Can you work these out from the model? Positions are in its coordinate system, mm. Face numbers are marked on the shaded views. A direction names the side the tool comes from. Coordinates: 2 decimals unless noted, no trailing zeros. Order: outer loops, then holes, each group sorted by start corner. A loop starts at its lowest first (then second) coordinate and runs counter-clockwise, first axis right, second up. Notation, with made-up numbers: M 46,-34 L 67,-34 A10 ccw 67,-23 Z; hole C 35,-22.75 d3. An arc over 180 degrees is marked long. Answer as a JSON object with one key per item and string values.
from build123d import *

# Parameters (mm, degrees)
SKETCH_4_W          = 28.4
SKETCH_4_H          = 61.796304386
EXTRUDE_1_DEPTH     = 5
CUT_EXTRUDE_START   = 5
SKETCH_4_4_R        = 3.1
CUT_EXTRUDE_1_DEPTH = 2.6
SKETCH_4_5_R        = 2
CUT_EXTRUDE_2_DEPTH = 74.193425166
SKETCH_4_6_W        = 13.4
SKETCH_4_6_H        = 41.796304386
CUT_EXTRUDE_3_DEPTH = 69.193425166
SKETCH_5_W          = 5
SKETCH_5_H          = 20
EXTRUDE_2_DEPTH     = 4
SKETCH_5_3_R        = 1.5
CUT_EXTRUDE_5_DEPTH = 69.193425166
CUT_EXTRUDE_START_2 = 4
SKETCH_5_4_R        = 2.25
CUT_EXTRUDE_7_DEPTH = 2


with BuildPart() as part:
    # 草图4 → 凸台-拉伸1 (new body)
    with BuildSketch(Plane(origin=(0, 0, 0), x_dir=(1, 0, 0), z_dir=(0, 1, 0))):
        with Locations((-14.2, -30.898152193)):
            Rectangle(SKETCH_4_W, SKETCH_4_H)
    extrude(amount=EXTRUDE_1_DEPTH)

    # 草图4<4> → 切除-拉伸1 (cut)
    with BuildSketch(Plane(origin=(0, 0, 0), x_dir=(1, 0, 0), z_dir=(0, 1, 0)).offset(CUT_EXTRUDE_START)):
        with Locations(Location((-13.9, -13.4, 0), (0, 0, 90))):
            Circle(SKETCH_4_4_R)
        with Locations(Location((-23.4, -34.346360066, 0), (0, 0, 90))):
            Circle(SKETCH_4_4_R)
        with Locations(Location((-18.4, -56.796304386, 0), (0, 0, 90))):
            Circle(SKETCH_4_4_R)
    extrude(amount=-CUT_EXTRUDE_1_DEPTH, mode=Mode.SUBTRACT)

    # 草图4<5> → 切除-拉伸2 (cut, through all)
    with BuildSketch(Plane(origin=(0, 0, 0), x_dir=(1, 0, 0), z_dir=(0, 1, 0)).offset(CUT_EXTRUDE_START)):
        with Locations(Location((-13.9, -13.4, 0), (0, 0, 90))):
            Circle(SKETCH_4_5_R)
        with Locations(Location((-23.4, -34.346360066, 0), (0, 0, 90))):
            Circle(SKETCH_4_5_R)
        with Locations(Location((-18.4, -56.796304386, 0), (0, 0, 90))):
            Circle(SKETCH_4_5_R)
    extrude(amount=-CUT_EXTRUDE_2_DEPTH, mode=Mode.SUBTRACT)

    # 草图4<6> → 切除-拉伸3 (cut, through all)
    with BuildSketch(Plane(origin=(0, 0, 0), x_dir=(1, 0, 0), z_dir=(0, 1, 0))):
        with Locations((-6.7, -40.898152193)):
            Rectangle(SKETCH_4_6_W, SKETCH_4_6_H)
    extrude(amount=CUT_EXTRUDE_3_DEPTH, mode=Mode.SUBTRACT)

    # 草图5 → 凸台-拉伸2 (add)
    with BuildSketch(Plane.XZ):
        Polygon((5, -10), (5, 20), (-28.4, 20), (-28.4, -10), (0, -10), align=None)
        with Locations((2.5, -20)):
            Rectangle(SKETCH_5_W, SKETCH_5_H)
    extrude(amount=EXTRUDE_2_DEPTH)

    # 草图5<3> → 切除-拉伸5 (cut, through all)
    with BuildSketch(Plane.XZ):
        with Locations(Location((-17.4, -5, 0), (0, 0, 270))):
            Circle(SKETCH_5_3_R)
        with Locations(Location((-5, -5, 0), (0, 0, 270))):
            Circle(SKETCH_5_3_R)
        with Locations(Location((2.5, 10, 0), (0, 0, 270))):
            Circle(SKETCH_5_3_R)
        with Locations(Location((2.5, -20, 0), (0, 0, 270))):
            Circle(SKETCH_5_3_R)
    extrude(amount=CUT_EXTRUDE_5_DEPTH, mode=Mode.SUBTRACT)

    # 草图5<4> → 切除-拉伸7 (cut)
    with BuildSketch(Plane.XZ.offset(CUT_EXTRUDE_START_2)):
        with Locations(Location((-17.4, -5, 0), (0, 0, 270))):
            Circle(SKETCH_5_4_R)
        with Locations(Location((-5, -5, 0), (0, 0, 270))):
            Circle(SKETCH_5_4_R)
        with Locations(Location((2.5, 10, 0), (0, 0, 270))):
            Circle(SKETCH_5_4_R)
        with Locations(Location((2.5, -20, 0), (0, 0, 270))):
            Circle(SKETCH_5_4_R)
    extrude(amount=-CUT_EXTRUDE_7_DEPTH, mode=Mode.SUBTRACT)


solid = part.part
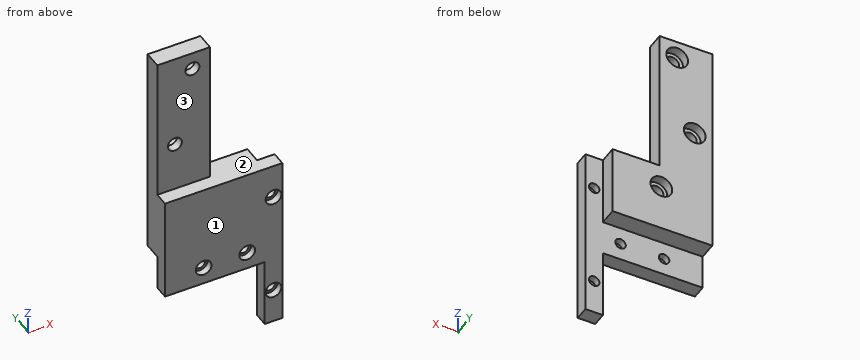
Item 1: I'm going to push flat-ended pins straight in: pin 1 (3 mm diameter, centred on x = -13, z = 14, fed in from +Y); pin 2 (2.5 mm diameter, centred on y = 1.5, z = 44.5, fed in from +X); pin 3 (1.2 mm diameter, centred on x = -14.5, z = 14, fed in from +Y). Where does each tip first touch, or does it pass through?
Answers follow:
{"pin 1": "stops at y = 2.4", "pin 2": "stops at x = -13.4", "pin 3": "stops at y = 0"}
Item 2: I want a section at D-D, the plane z = 40. Write out the boundary of the cut face in (x, y), plus the area to 3 significant figures.
Answers follow:
{"outline": "M -28.4,0 L -13.4,0 L -13.4,5 L -28.4,5 Z", "area": "75.0 mm^2"}
Item 3: I want a section at B-B, the plane y = 1. Write out the boundary of the cut face in (x, z), plus the area to 3 significant figures.
Answers follow:
{"outline": "M -28.4,0 L 0,0 L 0,20 L -13.4,20 L -13.4,61.8 L -28.4,61.8 Z; hole C -23.4,34.35 d4; hole C -18.4,56.8 d4; hole C -13.9,13.4 d4", "area": "1,160 mm^2"}
Item 4: I want a section at A-A, the plane z = -5. Write out the boundary of the cut face in (x, y), plus the area to 3 significant figures.
Answers follow:
{"outline": "M -28.4,-4 L -19.65,-4 L -19.65,-2 L -18.9,-2 L -18.9,0 L -28.4,0 Z; M -15.9,-2 L -15.15,-2 L -15.15,-4 L -7.25,-4 L -7.25,-2 L -6.5,-2 L -6.5,0 L -15.9,0 Z; M -3.5,-2 L -2.75,-2 L -2.75,-4 L 5,-4 L 5,0 L -3.5,0 Z", "area": "104 mm^2"}
Item 5: I want a section at C-C, the plane z = -20. Write out the boundary of the cut face in (x, y), plus the area to 3 significant figures.
Answers follow:
{"outline": "M 0,-4 L 0.25,-4 L 0.25,-2 L 1,-2 L 1,0 L 0,0 Z; M 4,-2 L 4.75,-2 L 4.75,-4 L 5,-4 L 5,0 L 4,0 Z", "area": "5.00 mm^2"}
Item 6: Which directions (+Z, -Z, +X, -X, +Y, -Y) give clear straight access to the entire face, cutting with the end or side of a thin tool? Please do the marked faces 1, 2 and 3.
Answers follow:
{"face 1": "+Z, -Z, +X, -X, -Y", "face 2": "+Z, +X, -Y", "face 3": "+Z, +X, -X, -Y"}
Item 7: Please list where these lines run through material, in increasing order: line 1 (X direction, y = -1.5, z = -5); line 2 (X direction, y = -3.2, z = -5); line 3 (Z direction, x = -23.4, y = 1.3).
Answers follow:
{"line 1": "x = -28.4 to -18.9, -15.9 to -6.5, -3.5 to 5", "line 2": "x = -28.4 to -19.65, -15.15 to -7.25, -2.75 to 5", "line 3": "z = 0 to 32.35, 36.35 to 61.8"}
